Autodesk Inventor part; units mm, degrees
ref_plane "YZ Plane" through (0, 0, 0) normal (1, 0, 0) x (0, 1, 0)
ref_plane "XZ Plane" through (0, 0, 0) normal (0, 1, 0) x (-1, 0, 0)
ref_plane "XY Plane" through (0, 0, 0) normal (0, 0, 1) x (1, 0, 0)
sketch "Skizze1" plane through (0, 0, 0) normal (0, 0, 1) x (1, 0, 0)
  circle A0 centre (0, 0) radius 19.4 construction
  circle A1 centre (0, 0) radius 9.75
  circle A2 centre (0, 19.4) radius 1.15
  line L0 (0, 0) -> (-16.8009, -9.7) construction
  line L1 (0, 34.057) -> (0, -28.3095) construction
  line L2 (-32.8873, 0) -> (32.8873, 0) construction
  circle A3 centre (0, 0) radius 6.35 construction
  circle A4 centre (0, 6.35) radius 1.5
  circle A5 centre (0, -6.35) radius 1.5
  circle A6 centre (6.35, 0) radius 1.5
  circle A7 centre (-6.35, 0) radius 1.5
  arc A8 (0, 24.55) -> (-4.46, 21.975) centre (0, 19.4) ccw
  circle A9 centre (16.8009, -9.7) radius 1.15
  arc A10 (16.8009, -14.85) -> (21.2609, -7.125) centre (16.8009, -9.7) ccw
  circle A11 centre (-16.8009, -9.7) radius 1.15
  arc A12 (-21.2609, -7.125) -> (-16.8009, -14.85) centre (-16.8009, -9.7) ccw
  circle A13 centre (0, 19.4) radius 2.85
  circle A14 centre (16.8009, -9.7) radius 2.85
  circle A15 centre (-16.8009, -9.7) radius 2.85
  circle A16 centre (0, 19.4) radius 4.5
  circle A17 centre (16.8009, -9.7) radius 4.5
  circle A18 centre (-16.8009, -9.7) radius 4.5
  line L3 (-4.46, 21.975) -> (-21.2609, -7.125)
  line L4 (-16.8009, -14.85) -> (16.8009, -14.85)
  line L5 (4.46, 21.975) -> (21.2609, -7.125)
  arc A19 (4.46, 21.975) -> (0, 24.55) centre (0, 19.4) ccw
  circle A20 centre (0, 19.4) radius 2.2 construction
  line L6 (1.2702, 21.6) -> (2.5403, 19.4)
  line L7 (2.5403, 19.4) -> (1.2702, 17.2)
  line L8 (1.2702, 17.2) -> (-1.2702, 17.2)
  line L9 (-1.2702, 17.2) -> (-2.5403, 19.4)
  line L10 (-2.5403, 19.4) -> (-1.2702, 21.6)
  line L11 (-1.2702, 21.6) -> (1.2702, 21.6)
  circle A21 centre (-16.8009, -9.7) radius 2.2 construction
  circle A22 centre (16.8009, -9.7) radius 2.2 construction
  line L12 (-18.0695, -11.9009) -> (-19.3412, -9.7018)
  line L13 (-19.3412, -9.7018) -> (-18.0726, -7.5009)
  line L14 (-18.0726, -7.5009) -> (-15.5322, -7.4991)
  line L15 (-15.5322, -7.4991) -> (-14.2606, -9.6982)
  line L16 (-14.2606, -9.6982) -> (-15.5292, -11.8991)
  line L17 (-15.5292, -11.8991) -> (-18.0695, -11.9009)
  line L18 (15.865, -12.0617) -> (14.2877, -10.0703)
  line L19 (14.2877, -10.0703) -> (15.2236, -7.7087)
  line L20 (15.2236, -7.7087) -> (17.7368, -7.3383)
  line L21 (17.7368, -7.3383) -> (19.3141, -9.3297)
  line L22 (19.3141, -9.3297) -> (18.3782, -11.6913)
  line L23 (18.3782, -11.6913) -> (15.865, -12.0617)
  point P0 (0, 21.6)
  point P1 (-16.8009, -9.7)
  point P2 (-16.7994, -11.9)
  point P3 (17.1216, -11.8765)
  dimension "d31" = 4.4
  dimension "d0" = 38.8
  dimension "d1" = 2.3
  dimension "d2" = 30
  dimension "d3" = 19.5
  dimension "d4" = 12.7
  dimension "d5" = 3
  dimension "d8" = 4
  dimension "d26" = 5.7
  dimension "d30" = 9
extrude "Extrusion1" add sketch "Skizze1" along normal blind 3 contours A1 | A19 L5 A10 L4 A12 L3 A8 | A13 | A14 | A15 | A16 | A17 | A18 | L6 L7 L8 L9 L10 L11 | L12 L13 L14 L15 L16 L17 | L18 L19 L20 L21 L22 L23
extrude "Extrusion3" cut sketch "Skizze1" along normal blind 1.5 contours A1
extrude "Extrusion4" add sketch "Skizze1" along normal blind 3 from surface at 3 contours A13 | A14 | A15 | A16 | A17 | A18 | L6 L7 L8 L9 L10 L11 | L12 L13 L14 L15 L16 L17 | L18 L19 L20 L21 L22 L23
extrude "Extrusion6" add sketch "Skizze1" along normal blind 3 from surface at 6 contours A13 | A14 | A15 | L6 L7 L8 L9 L10 L11 | L12 L13 L14 L15 L16 L17 | L18 L19 L20 L21 L22 L23
extrude "Extrusion8" cut sketch "Skizze1" along normal blind 1.5 contours L6 L7 L8 L9 L10 L11 | L12 L13 L14 L15 L16 L17 | L18 L19 L20 L21 L22 L23
properties part number "PlanetaryHolderTop"
Model file for the job. Use its own axes, mm. A direction names the side the tool comes from. Coordinates: 2 decimals unless noted, no trailing zeros. Write each loop counter-clockwise with the first axis right and the second up, starting at its lowest first coordinate (ties: lowest second). Pieces come first, ordered by that corner, then holes. Notation, with made-up numbers: (45.25, -1) - (71.25, -1) arc R11 cw to (71.25, 11) - close; hole circle Ø4 at (-6, 45.5). An arc over 180 degrees is marked (long way). Use a Markdown table: item, result. Add a question column.
Item 1: Two-plate mould, pull along Y, no slides. Class faces 4 (the face through (17.139, -11.874, 0.74)), 5 (the face through (13.954, -9.825, 7.479)), 6 (the face through (0, 1, 3)): pulls with the +Y half, pulls with the -Y half, needs draft (parallel to the pull), parting line crosses it, or undercut.
Item 2: 3-axis set-ups, long thin cutter, end or side, ignore diameter. For faces 1 (the face through (-2.61, 23.84, 1.48)), 2 (the face through (0, 0, 1.5)), 3 (the face through (-0.62, 22.18, 7.48)): which of +Z, -Z, +X, -X, +Y, -Y reach the whole face in a straight line?
Item 3: Drop flat-ended pins along their axis: pin 1 (8 mm diameter, centred on x = 8, y = -1, fed in from -Z); pin 2 (1 mm diameter, centred on x = 13.5, z = 6, fed in from +Y); pin 3 (3 mm diameter, centred on x = -5, y = 14, fed in from +Z); pin 4 (3.5 mm diameter, centred on x = -6.35, y = 0, fed in from -Z). Give the stop position or say it passes through.
Item 4: Band-saw the part on B-B, the plane y = 0. Write the cut outline in (x, z).
Item 5: Band-saw the part on A-A, the plane z = 7.25. Write the cut outline in (x, y), and give its area (3 significant figures).
Item 6: Drill centre lines: line 1 along Y through (x, z) = (0, 1); line 2 along Y through (x, z) = (2, 1); line 3 along Z through (x, y) = (-5.5, 18.5). Where is each one in solid material? Low to high.
Item 7: Band-saw the part on D-D, the plane y = 6.35. Write the cut outline in (x, z), and give its area (3 significant figures).
Item 8: Band-saw the part on C-C, the plane x = -6.35. Write the cut outline in (y, z), and give its area (3 significant figures).
A:
| question | item | result |
|---|---|---|
| 1 | face 4 | undercut |
| 1 | face 5 | parting line crosses it |
| 1 | face 6 | needs draft |
| 2 | face 1 | +Z, -Z, -X, +Y |
| 2 | face 2 | -Z |
| 2 | face 3 | +Z |
| 3 | pin 1 | stops at z = 0 |
| 3 | pin 2 | stops at y = -6.18 |
| 3 | pin 3 | stops at z = 3 |
| 3 | pin 4 | stops at z = 1.5 |
| 4 | outline | (-17.15, 0) - (-9.75, 0) - (-9.75, 1.5) - (-7.85, 1.5) - (-7.85, 3) - (-17.15, 3) - close; (-4.85, 1.5) - (4.85, 1.5) - (4.85, 3) - (-4.85, 3) - close; (7.85, 1.5) - (9.75, 1.5) - (9.75, 0) - (17.15, 0) - (17.15, 3) - (7.85, 3) - close |
| 5 | outline | circle Ø5.7 at (-16.8, -9.7); circle Ø5.7 at (0, 19.4); circle Ø5.7 at (16.8, -9.7); hole circle Ø2.3 at (-16.8, -9.7); hole circle Ø2.3 at (0, 19.4); hole circle Ø2.3 at (16.8, -9.7) |
| 5 | area | 64.1 mm² |
| 6 | line 1 | y = -14.85 to -9.75, 9.75 to 17.2, 21.6 to 24.55 |
| 6 | line 2 | y = -14.85 to -9.54, 9.54 to 18.46, 20.34 to 24.15 |
| 6 | line 3 | z = 0 to 3 |
| 7 | outline | (-13.48, 0) - (-7.4, 0) - (-7.4, 1.5) - (-1.5, 1.5) - (-1.5, 3) - (-13.48, 3) - close; (1.5, 1.5) - (7.4, 1.5) - (7.4, 0) - (13.48, 0) - (13.48, 3) - (1.5, 3) - close |
| 7 | area | 54.2 mm² |
| 8 | outline | (-14.85, 0) - (-7.4, 0) - (-7.4, 1.5) - (-1.5, 1.5) - (-1.5, 3) - (-14.85, 3) - close; (1.5, 1.5) - (7.4, 1.5) - (7.4, 0) - (18.7, 0) - (18.7, 3) - (1.5, 3) - close |
| 8 | area | 74.0 mm² |
